```python
from build123d import *

# Parameters (mm, degrees)
SKETCH1_R           = 96.5
SKETCH1_R_2         = 39
BOSS_EXTRUDE1_DEPTH = 5.8
SKETCH2_R           = 58.5
SKETCH2_R_2         = 51.5
CUT_EXTRUDE1_DEPTH  = 3.5
SKETCH3_R           = 2
CUT_EXTRUDE2_DEPTH  = 6.8


with BuildPart() as part:
    # Sketch1 → Boss-Extrude1 (new body)
    with BuildSketch(Plane(origin=(0, 0, 0), x_dir=(1, 0, 0), z_dir=(0, 1, 0))):
        Circle(SKETCH1_R)
        Circle(SKETCH1_R_2, mode=Mode.SUBTRACT)
    extrude(amount=BOSS_EXTRUDE1_DEPTH)

    # Sketch2 → Cut-Extrude1 (cut)
    with BuildSketch(Plane(origin=(0, 5.8, 0), x_dir=(1, 0, 0), z_dir=(0, 1, 0))):
        Circle(SKETCH2_R)
        Circle(SKETCH2_R_2, mode=Mode.SUBTRACT)
    extrude(amount=-CUT_EXTRUDE1_DEPTH, mode=Mode.SUBTRACT)

    # Sketch3 → Cut-Extrude2 (cut, through all)
    with BuildSketch(Plane(origin=(0, 5.8, 0), x_dir=(1, 0, 0), z_dir=(0, 1, 0))):
        with Locations((0, 86.5)):
            Circle(SKETCH3_R)
        with Locations((74.911197427, 43.25)):
            Circle(SKETCH3_R)
        with Locations((74.911197427, -43.25)):
            Circle(SKETCH3_R)
        with Locations((0, -86.5)):
            Circle(SKETCH3_R)
        with Locations((-74.911197427, -43.25)):
            Circle(SKETCH3_R)
        with Locations((-74.911197427, 43.25)):
            Circle(SKETCH3_R)
    extrude(amount=-CUT_EXTRUDE2_DEPTH, mode=Mode.SUBTRACT)


solid = part.part
```
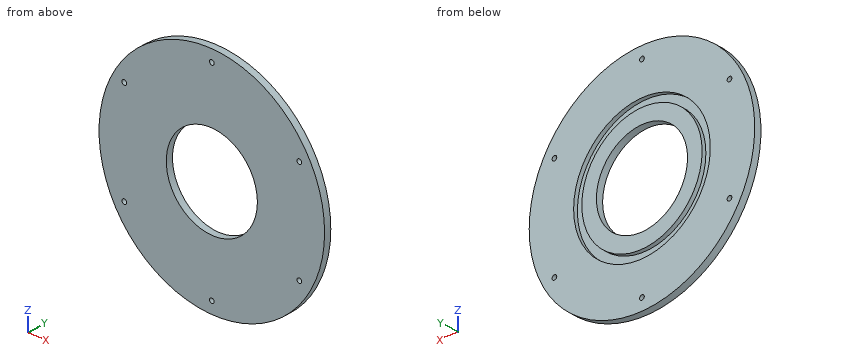
Could you check a few things on this model? Use its own coordinates, in mm. Coordinates: 2 decimals unless noted, no trailing zeros. Loops run counter-clockwise (first coordinate to the right, second up) from the corner with the lowest first, then second, coordinate; pieces in that order, holes last.
1) Will these pins go through, and if not, where does the flat tip stop? pin 1 Ø1.5 at (x, z) = (-19, 53.5) entering from -Y; pin 2 Ø2 at (x, y) = (65.5, 1.5) entering from -Z; pin 3 Ø1.5 at (x, z) = (-27, -49.5) entering from +Y; pin 4 Ø1 at (y, z) = (4.5, 55) entering from -X.
Reported:
pin 1: stops at y = 0
pin 2: stops at z = -71.78
pin 3: stops at y = 2.3
pin 4: stops at x = -79.64
2) Imagine slicing it at B-B (y = 3.45). State how many separate pieces and enclosed holes the cut face has, and give its area (3 significant figures).
Reported:
separate pieces: 2
enclosed holes: 8
area: 22,000 mm2
3) Imagine slicing it at D-D (x = -66). List the corners of the cut face in (y, z) for me, and give its area (3 significant figures).
Reported:
outline: (0, -70.4) - (5.8, -70.4) - (5.8, 70.4) - (0, 70.4) - close
area: 817 mm2
4) Imagine slicing it at C-C (x = 14.5). List the corners of the cut face in (y, z) for me.
Reported:
outline: (0, -95.4) - (5.8, -95.4) - (5.8, -56.67) - (2.3, -56.67) - (2.3, -49.42) - (5.8, -49.42) - (5.8, -36.2) - (0, -36.2) - close; (0, 36.2) - (5.8, 36.2) - (5.8, 49.42) - (2.3, 49.42) - (2.3, 56.67) - (5.8, 56.67) - (5.8, 95.4) - (0, 95.4) - close
5) Imagine slicing it at A-A (z = 0). List the corners of the cut face in (x, y) for me, and give its area (3 significant figures).
Reported:
outline: (-96.5, 0) - (-39, 0) - (-39, 5.8) - (-51.5, 5.8) - (-51.5, 2.3) - (-58.5, 2.3) - (-58.5, 5.8) - (-96.5, 5.8) - close; (39, 0) - (96.5, 0) - (96.5, 5.8) - (58.5, 5.8) - (58.5, 2.3) - (51.5, 2.3) - (51.5, 5.8) - (39, 5.8) - close
area: 618 mm2
6) Please list where these lines run through material, in increasing order: line 1 along Z through (x, y) = (0, 2.65); line 2 along X through (y, z) = (3.75, 0); line 3 along X through (y, z) = (2.2, -43.25).
Reported:
line 1: z = -96.5 to -88.5, -84.5 to -58.5, -51.5 to -39, 39 to 51.5, 58.5 to 84.5, 88.5 to 96.5
line 2: x = -96.5 to -58.5, -51.5 to -39, 39 to 51.5, 58.5 to 96.5
line 3: x = -86.27 to -76.91, -72.91 to 72.91, 76.91 to 86.27
